```python
from build123d import *

# Parameters (mm, degrees)
SKETCH1_W               = 163
SKETCH1_H               = 10
BOSS_EXTRUDE1_DEPTH     = 20
SKETCH4_W               = 120
SKETCH4_H               = 20
BOSS_EXTRUDE2_DEPTH     = 5.84
CUT_EXTRUDE1_REACH      = 86.512
SKETCH5_W               = 100
SKETCH5_H               = 5
CUT_EXTRUDE2_DEPTH      = 10
CUT_EXTRUDE3_DEPTH      = 86.399974239
CUT_EXTRUDE3_DEPTH_BACK = 86.399974239
SKETCH2_R               = 1.75
SKETCH7_W               = 8
SKETCH7_H               = 15.84
BOSS_EXTRUDE3_DEPTH     = 2


with BuildPart() as part:
    # Sketch1 → Boss-Extrude1 (new body)
    with BuildSketch(Plane.XY):
        with Locations((0, 5)):
            Rectangle(SKETCH1_W, SKETCH1_H)
    extrude(amount=BOSS_EXTRUDE1_DEPTH)

    # Sketch4 → Boss-Extrude2 (add)
    with BuildSketch(Plane.XZ):
        with Locations((0, 10)):
            Rectangle(SKETCH4_W, SKETCH4_H)
        with BuildLine():
            Line((-45, 12.35), (45, 12.35))
            ThreePointArc((45, 12.35), (47.35, 10), (45, 7.65))
            Line((45, 7.65), (-45, 7.65))
            ThreePointArc((-45, 7.65), (-47.35, 10), (-45, 12.35))
        make_face(mode=Mode.SUBTRACT)
    extrude(amount=BOSS_EXTRUDE2_DEPTH)

    # Cut-Extrude1: up to this face of the body (flat: up to its plane)
    cut_extrude1_end = Plane(part.part.faces().sort_by_distance((0, 2.618699159, 0))[0])
    # Sketch5 → Cut-Extrude1 (cut, up to the picked face)
    with BuildSketch(Plane.XY.offset(20), mode=Mode.PRIVATE) as cut_extrude1_sk1:
        with Locations((0, -0.34)):
            Rectangle(SKETCH5_W, SKETCH5_H)
    cut_extrude1_tool1 = split(extrude(cut_extrude1_sk1.sketch, amount=-CUT_EXTRUDE1_REACH, mode=Mode.PRIVATE), bisect_by=cut_extrude1_end, keep=Keep.BOTH, mode=Mode.PRIVATE)
    add(cut_extrude1_tool1.solids().sort_by(Axis((0, -0.34, 20), (0, 0, -1)))[0], mode=Mode.SUBTRACT)

    # Sketch6 → Cut-Extrude2 (cut)
    with BuildSketch(Plane.XZ.offset(-2.16)):
        with BuildLine():
            Line((-45, 5), (45, 5))
            ThreePointArc((45, 5), (50, 10), (45, 15))
            Line((45, 15), (-45, 15))
            ThreePointArc((-45, 15), (-50, 10), (-45, 5))
        make_face()
    extrude(amount=-CUT_EXTRUDE2_DEPTH, mode=Mode.SUBTRACT)

    # Sketch2 → Cut-Extrude3 (cut, two sides: drawn at the far end of the back side and taken through both)
    with BuildSketch(Plane(origin=(0, 10, 0), x_dir=(1, 0, 0), z_dir=(0, 1, 0)).offset(-CUT_EXTRUDE3_DEPTH_BACK)):
        with Locations(Location((76.5, -10, 0), (0, 0, 180))):
            Circle(SKETCH2_R)
        with Locations(Location((-76.5, -10, 0), (0, 0, 180))):
            Circle(SKETCH2_R)
    extrude(amount=CUT_EXTRUDE3_DEPTH + CUT_EXTRUDE3_DEPTH_BACK, mode=Mode.SUBTRACT)

    # Sketch7 → Boss-Extrude3 (add)
    with BuildSketch(Plane.XY.offset(20)):
        with Locations((-15, 2.08)):
            Rectangle(SKETCH7_W, SKETCH7_H)
        with Locations((15, 2.08)):
            Rectangle(SKETCH7_W, SKETCH7_H)
    extrude(amount=BOSS_EXTRUDE3_DEPTH)


solid = part.part
```
Geometry check sheet. Reference: the model listing, model coordinates, mm. A direction names the side the tool comes from. Coordinates: 2 decimals unless noted, no trailing zeros. Order: outer loops, then holes, each group sorted by start corner. A loop starts at its lowest first (then second) coordinate and runs counter-clockwise, first axis right, second up. Notation, with made-up numbers: M 24.25,-1 L 59.25,-1 A24 ccw 59.25,17 Z; hole C -2,87 d6. An arc over 180 degrees is marked long. Answer as a JSON object with one key per item and string values.
Q1. Cross-section at B-B on y = 5.5. Record the cut outline in (x, z), and give its area (3 significant figures).
Results are:
{"outline": "M -81.5,0 L 81.5,0 L 81.5,20 L 19,20 L 19,22 L 11,22 L 11,20 L -11,20 L -11,22 L -19,22 L -19,20 L -81.5,20 Z; hole C -76.5,10 d3.5; hole M -45,5 L 45,5 A5 ccw 45,15 L -45,15 A5 ccw Z; hole C 76.5,10 d3.5", "area": "2,290 mm²"}
Q2. Release check for a two-part mould opening along Z. For faces 5 (the flat face through (-15, 0, 20)), 6 (the flat face through (60, -3, 10)), 7 (the cylindrical face through (74.831, 4.93, 10.526)) record: released by +Z, released by -Z, zero draft, split by the parting line, or undercut.
Results are:
{"face 5": "released by -Z", "face 6": "zero draft", "face 7": "undercut"}
Q3. Cross-section at D-D on x = -57.5. Record the cut outline in (y, z), and give its area (3 significant figures).
Results are:
{"outline": "M -5.84,0 L 10,0 L 10,20 L -5.84,20 Z", "area": "317 mm²"}
Q4. Scan lines: line 1 (X direction, y = 4.25, z = 10); line 2 (Z direction, x = -76.5, y = 3); line 3 (Y direction, x = -2, z = 17). Record each from-to range of solid material in increasing order.
Results are:
{"line 1": "x = -81.5 to -78.25, -74.75 to -50, 50 to 74.75, 78.25 to 81.5", "line 2": "z = 0 to 8.25, 11.75 to 20", "line 3": "y = -5.84 to -2.84, 2.16 to 10"}
Q5. Cross-section at A-A on x = 76.5. Record the cut outline in (y, z).
Results are:
{"outline": "M 0,0 L 10,0 L 10,8.25 L 0,8.25 Z; M 0,11.75 L 10,11.75 L 10,20 L 0,20 Z"}
Q6. Tool access check on faces 1 (the cylindrical face through (47.35, -4.32, 10.05)), 2 (the cylindrical face through (-50, 6, 10)), 3 (the flat face through (-51, 4, 20)), 4 (the flat face through (71, 0, 10)). Record the directions out of +Z, -Z, +X, -X, +Y, -Y that give a thin tool (end or side, any length) a straight path to the whole face; none if there is none.
Results are:
{"face 1": "+Y, -Y", "face 2": "+Y", "face 3": "+Z, -X, +Y, -Y", "face 4": "+Z, -Z, +X, -Y"}
Q7. Depth check by flat-ended pin: pin 1 Ø1 at (y, z) = (-1.5, 21.5) entering from +X; pin 2 Ø10 at (x, z) = (76, 14.5) entering from -Y; pin 3 Ø1.5 at (x, y) = (-62, 2) entering from +Z; pin 4 Ø2 at (x, z) = (-76.5, 10) entering from -Y. Enter the tip coordinate at first touch or a pass-through.
Results are:
{"pin 1": "stops at x = 19", "pin 2": "stops at y = 0", "pin 3": "stops at z = 20", "pin 4": "passes through"}
Q8. Cross-section at C-C on x = 34. Record the cut outline in (y, z).
Results are:
{"outline": "M -5.84,0 L -2.84,0 L -2.84,7.65 L -5.84,7.65 Z; M -5.84,12.35 L -2.84,12.35 L -2.84,20 L -5.84,20 Z; M 2.16,0 L 10,0 L 10,5 L 2.16,5 Z; M 2.16,15 L 10,15 L 10,20 L 2.16,20 Z"}
